Could you check a few things on this model? Use its own coordinates, in mm. A direction names the side the tool comes from. Give positions to 0.01 mm unless a question says otherwise; leave off trailing zeros. Write each loop counter-clockwise with the first axis right and the second up, starting at its lowest first coordinate (ties: lowest second). Pieces come first, ordered by that corner, then holes. Notation, with made-up numbers: M 45.25,43.25 L 88.25,43.25 A11 cw 88.25,62.25 Z; hole C -10,13 d6. An arc over 180 degrees is marked long. Use one line per item in the form item = value.
Autodesk Inventor part; units mm, degrees
ref_plane "YZ Plane" through (0, 0, 0) normal (1, 0, 0) x (0, 1, 0)
ref_plane "XZ Plane" through (0, 0, 0) normal (0, 1, 0) x (-1, 0, 0)
ref_plane "XY Plane" through (0, 0, 0) normal (0, 0, 1) x (1, 0, 0)
sketch "Sketch1" plane through (0, 0, 0) normal (0, 0, 1) x (1, 0, 0)
  circle A0 centre (0, 0) radius 3
  dimension "d0" = 6
extrude "Extrusion1" add sketch "Sketch1" along normal blind 3
sketch "Sketch5" plane through (0, 0, 3) normal (0, 0, 1) x (1, 0, 0)
  circle A0 centre (0, 0) radius 1.5
  dimension "d6" = 3
extrude "Extrusion3" add sketch "Sketch5" along normal blind 5
sketch "Sketch6" plane through (0, 0, 8) normal (0, 0, 1) x (1, 0, 0)
  circle A0 centre (0, 0) radius 1
  dimension "d9" = 2
extrude "Extrusion4" add sketch "Sketch6" along normal blind 3
sketch "Sketch7" plane through (0, 0, 11) normal (0, 0, 1) x (1, 0, 0)
  circle A0 centre (0, 0) radius 1
  circle A1 centre (0, 0) radius 1.5
  dimension "d12" = 3
extrude "Extrusion5" add sketch "Sketch7" along normal blind 50 contours A0 | A1
sketch "Sketch8" plane through (0, 0, 61) normal (0, 0, 1) x (1, 0, 0)
  circle A0 centre (0, 0) radius 1
  dimension "d15" = 2
extrude "Extrusion6" add sketch "Sketch8" along normal blind 3
sketch "Sketch9" plane through (0, 0, 64) normal (0, 0, 1) x (1, 0, 0)
  circle A0 centre (0, 0) radius 1.5
  dimension "d18" = 3
extrude "Extrusion7" add sketch "Sketch9" along normal blind 5
sketch "Sketch10" plane through (0, 0, 69) normal (0, 0, 1) x (1, 0, 0)
  circle A0 centre (0, 0) radius 1
  circle A1 centre (0, 0) radius 1
  dimension "d21" = 2
extrude "Extrusion8" add sketch "Sketch10" along normal blind 3
sketch "Sketch11" plane through (0, 0, 72) normal (0, 0, 1) x (1, 0, 0)
  circle A0 centre (0, 0) radius 1.5
  circle A1 centre (0, 0) radius 1.5
  dimension "d24" = 3
extrude "Extrusion9" add sketch "Sketch11" along normal blind 5
properties part number "TornilloBasePixhawx"
1) I want a section at C-C, the plane z = 32.5. Please give me the cut outline in (x, y).
Checked values:
outline = C 0,0 d3
2) For faces 5 (the cylindrical face through (-3, 0, 1)), 6 (the cylindrical face through (-1.5, -0.07, 5.46)), 7 (the cylindrical face through (0, 1, 62)), which set-ups out of +Z, -Z, +X, -X, +Y, -Y let a thin tool reach every point of the face, with its end or its side?
Checked values:
face_5 = +Z, -Z
face_6 = +Z
face_7 = none
3) If I drill on L1, parallel to Z at x = -2.6, y = -0.4; L2, parallel to X at y = 0.2, z = 47; L3, parallel to Y at x = -0.05, z = 11.5, over which ranges is the centre line in solid material (lowest first)?
Checked values:
L1 = 0 to 3
L2 = -1.49 to 1.49
L3 = -1.5 to 1.5
4) For pin 1 Ø2 at (y, z) = (-0.5, 59.5) entering from +X; pin 2 Ø1.5 at (x, z) = (0, 11) entering from -Y; pin 3 Ø3.5 at (x, y) = (-0.5, 0.5) entering from -Z; pin 4 Ø1 at (y, z) = (-1.5, 8) entering from -X, each with a flat end and sliding along its axis, tell me the tip position at first contact or that it passes through.
Checked values:
pin_1 = 1.5
pin_2 = -1.5
pin_3 = 0
pin_4 = -1.12
5) Thinking about a two-plate mould opening in Z: for faces 1 (the flat face through (0, 0, 77)), 2 (the cylindrical face through (0, 1, 9)), 3 (the cylindrical face through (0, 1, 70)), 4 (the cylindrical face through (-1.5, -0.07, 66.46)), which applies, released by +Z, released by -Z, zero draft, split by the parting line, or undercut?
Checked values:
face_1 = released by +Z
face_2 = undercut
face_3 = undercut
face_4 = zero draft
